Design review of the part built by this model. Coordinates are the model's own, in mm. A direction names the side the tool comes from. Coordinates: 2 decimals unless noted, no trailing zeros. Write each loop counter-clockwise with the first axis right and the second up, starting at its lowest first coordinate (ties: lowest second). Pieces come first, ordered by that corner, then holes. Notation, with made-up numbers: M 77,-17.75 L 87,-17.75 A27 cw 87,2.25 Z; hole C 51.5,62.25 d11. An arc over 180 degrees is marked long. Write item = value, one per line.
```python
from build123d import *

# Parameters (mm, degrees)
BOSS_EXTRUDE1_DEPTH     = 170.18
CUT_EXTRUDE_THIN2_DEPTH = 3.81
CUT_EXTRUDE1_DEPTH      = 25.4
SKETCH4_R               = 1.4224
CUT_EXTRUDE2_DEPTH      = 10.16
SKETCH5_W               = 109.403315499
SKETCH5_H               = 17.948067256
CUT_EXTRUDE3_DEPTH      = 12.7
SKETCH6_R               = 1.905
CUT_EXTRUDE4_DEPTH      = 12.7


with BuildPart() as part:
    # Sketch1 → Boss-Extrude1 (new body)
    with BuildSketch(Plane.XY):
        Polygon((0, 139.7), (117.222218475, 0), (127.878783791, 0), (0, 152.4), align=None)
    extrude(amount=BOSS_EXTRUDE1_DEPTH)

    # Sketch2 → Cut-Extrude-Thin2 (cut)
    with BuildSketch(Plane(origin=(75.04235078, 62.968008862, 0), x_dir=(0, 0, -1), z_dir=(0.7660444431189745, 0.6427876096865436, 0))):
        Polygon((-137.16, -77.261258255), (-161.29, 108.554672373), (-156.252299153, 109.208866666), (-132.122299153, -76.607063962), align=None)
        Polygon((-33.02, -77.261258255), (-12.813831453, 108.554672373), (-7.763603235, 108.005495764), (-27.969771782, -77.810434864), align=None)
    extrude(amount=-CUT_EXTRUDE_THIN2_DEPTH, mode=Mode.SUBTRACT)

    # Sketch3 → Cut-Extrude1 (cut)
    with BuildSketch(Plane(origin=(75.04235078, 62.968008862, 0), x_dir=(0, 0, -1), z_dir=(0.7660444431189745, 0.6427876096865436, 0))):
        Polygon((-164.926611636, 9.038106978), (-164.926611636, -99.720446986), (-141.126263261, -99.720446986), (-155.587234425, 9.038106978), align=None)
        Polygon((-13.086414412, 9.038106978), (-27.246115343, -99.720446986), (-4.650847899, -99.720446986), (-4.650847899, 9.038106978), align=None)
    extrude(amount=-CUT_EXTRUDE1_DEPTH, mode=Mode.SUBTRACT)

    # Sketch4 → Cut-Extrude2 (cut)
    with BuildSketch(Plane.XY.offset(170.18)):
        with Locations((24.589669417, 116.745173131)):
            Circle(SKETCH4_R)
        with Locations((57.243279989, 77.830115421)):
            Circle(SKETCH4_R)
        with Locations((89.896890561, 38.91505771)):
            Circle(SKETCH4_R)
    cut_extrude2 = extrude(amount=-CUT_EXTRUDE2_DEPTH, mode=Mode.SUBTRACT)

    # Mirror1: Cut-Extrude2 across plane
    add(cut_extrude2.mirror(Plane.XY.offset(85.09)), mode=Mode.SUBTRACT)

    # Sketch5 → Cut-Extrude3 (cut)
    with BuildSketch(Plane(origin=(75.04235078, 62.968008862, 0), x_dir=(0, 0, -1), z_dir=(0.7660444431189746, 0.6427876096865437, 0))):
        with Locations((-83.900833528, -73.224864135)):
            Rectangle(SKETCH5_W, SKETCH5_H)
    extrude(amount=-CUT_EXTRUDE3_DEPTH, mode=Mode.SUBTRACT)

    # Sketch6 → Cut-Extrude4 (cut)
    with BuildSketch(Plane(origin=(72.123721451, 60.518988069, 0), x_dir=(0, 0, -1), z_dir=(0.7660444431189746, 0.6427876096865437, 0))):
        with Locations(Location((-154.682435242, 77.396139224, 0), (0, 0, 90))):
            Circle(SKETCH6_R)
        with Locations(Location((-138.327577907, -48.546381958, 0), (0, 0, 90))):
            Circle(SKETCH6_R)
        with Locations(Location((-13.719119266, 76.715945514, 0), (0, 0, 90))):
            Circle(SKETCH6_R)
        with Locations(Location((-27.440726954, -49.540608702, 0), (0, 0, 90))):
            Circle(SKETCH6_R)
    extrude(amount=-CUT_EXTRUDE4_DEPTH, mode=Mode.SUBTRACT)


solid = part.part
```
Q1. Consider section D-D, the plane y = 107. State the section outline as (x, z) points, and give its area (3 significant figures).
Check result:
outline = M 27.44,0 L 38.1,0 L 38.1,13.26 L 33.12,12.91 L 33.12,18.02 L 38.1,18.37 L 38.1,149.53 L 33.12,149.95 L 33.12,155.07 L 38.1,154.66 L 38.1,170.18 L 27.44,170.18 Z
area = 1,760 mm²
Q2. Machinability: for faces 4 (the cylindrical face through (101.193, 22.537, 26.711)), 5 (the flat face through (95.883, 31.87, 149.437)), 6 (the flat face through (58.374, 79.911, 145.147)), which of the approach directions +Z, -Z, +X, -X, +Y, -Y give a long, thin tool a straight path to every point of the face, cutting with its end or side? Answer none if there is none.
Check result:
face_4 = none
face_5 = +X, -Y
face_6 = +X
Q3. Consider section A-A, the plane x = 72. State the section outline as (y, z) points, and give its area (3 significant figures).
Check result:
outline = M 53.89,0 L 66.59,0 L 66.59,4.65 L 53.89,4.65 Z; M 53.89,14.91 L 66.59,13.65 L 66.59,18.99 L 60.67,19.49 L 60.67,24.6 L 66.59,24.1 L 66.59,142.69 L 60.67,142.1 L 60.67,147.22 L 66.59,147.81 L 66.59,155.01 L 53.89,153.72 Z; M 53.89,164.93 L 66.59,164.93 L 66.59,170.18 L 53.89,170.18 Z
area = 1,840 mm²
Q4. The part is to be moulded in two halves that separate along Y. For faces 1 (the flat face through (59, 71, 0)), 2 (the flat face through (60.14, 77.8, 22.34)), 3 (the flat face through (122, 0, 168)), say which applies: +Y half, -Y half, draft (parallel to the pull), parting line (faces both ways), or undercut.
Check result:
face_1 = draft
face_2 = undercut
face_3 = -Y half
Q5. Consider section B-B, the plane x = 11. State the section outline as (y, z) points, and give its area (3 significant figures).
Check result:
outline = M 126.59,0 L 139.29,0 L 139.29,8.67 L 133.36,9.17 L 133.36,14.28 L 139.29,13.78 L 139.29,155.01 L 133.36,154.42 L 133.36,159.54 L 139.29,160.13 L 139.29,170.18 L 126.59,170.18 Z
area = 2,100 mm²
Q6. Wall thickness on line 1 (Y direction, x = 39, z = 129.5); line 2 (X direction, y = 11.5, z = 54); line 3 (X direction, y = 86, z = 98.5): over which ranges is each line inside the solid? List them lowest first.
Check result:
line_1 = 93.22 to 105.92
line_2 = 107.57 to 113.66
line_3 = 45.06 to 55.72
Q7. Consider section C-C, the plane z = 81. State the section outline as (x, y) points.
Check result:
outline = M 0,139.7 L 110.09,8.5 L 116.34,13.75 L 0,152.4 Z
Q8. For P1, Ø3.5, axis at x = 57.24, y = 77.83, coming from the -Z side; P2, Ø10, axis at y = 44, z = 17, coming from the +X side; P3, Ø12, axis at x = 90.5, z = 133.5, coming from the -Y side; P4, Ø2.5, axis at x = 57.24, y = 77.83, coming from the +Z side, all flat-tipped, find the tip position at first contact; note any pin that passes through.
Check result:
P1 = 0
P2 = 95.01
P3 = 24.7
P4 = 160.02
